Here's how the part is built. I have some questions about the finished solid (model axes, mm). A direction names the side the tool comes from. Round coordinates to 2 decimals unless told otherwise and drop trailing zeros. Loops run counter-clockwise (first coordinate to the right, second up) from the corner with the lowest first, then second, coordinate; pieces in that order, holes last. Notation, with made-up numbers: (-10, 81) -> (24, 81) arc R25 cw to (24, 116) -> close; hole circle Ø8 at (-10, 30). An arc over 180 degrees is marked (long way). Use CSV: the item, a comma, the result in double quotes. Start each with the question number.
from build123d import *

# Parameters (mm, degrees)
EXTRUDE_1_DEPTH     = 15
SKETCH_2_R          = 3.25
SKETCH_2_W          = 10
SKETCH_2_H          = 7
CUT_EXTRUDE_1_DEPTH = 37
SKETCH_3_W          = 7
SKETCH_3_H          = 25
CUT_EXTRUDE_2_DEPTH = 37
FILLET_1_R          = 2
FILLET_2_R          = 2


with BuildPart() as part:
    # 草图1 → 凸台-拉伸1 (new body)
    with BuildSketch(Plane.XY):
        Polygon((-3.257989732, 3.83894099), (16.742010268, 3.83894099), (16.742010268, 0.83894099), (-18.257989732, 0.83894099), (-18.257989732, 24.83894099), (-3.257989732, 24.83894099), align=None)
        with BuildLine():
            Line((-12.257989732, 18.83894099), (-12.257989732, 8.83894099))
            ThreePointArc((-12.257989732, 8.83894099), (-10.757989732, 7.33894099), (-9.257989732, 8.83894099))
            Line((-9.257989732, 8.83894099), (-9.257989732, 18.83894099))
            ThreePointArc((-9.257989732, 18.83894099), (-10.757989732, 20.33894099), (-12.257989732, 18.83894099))
        make_face(mode=Mode.SUBTRACT)
    extrude(amount=EXTRUDE_1_DEPTH)

    # 草图2 → 切除-拉伸1 (cut)
    with BuildSketch(Plane(origin=(0, 24.83894099, 0), x_dir=(1, 0, 0), z_dir=(0, 1, 0))):
        with Locations(Location((6.742010268, -7.5, 0), (0, 0, 180))):
            Circle(SKETCH_2_R)
        with Locations((-13.257989732, -7.5)):
            Rectangle(SKETCH_2_W, SKETCH_2_H)
    extrude(amount=-CUT_EXTRUDE_1_DEPTH, mode=Mode.SUBTRACT)

    # 草图3 → 切除-拉伸2 (cut)
    with BuildSketch(Plane(origin=(-3.257989732, 0, 0), x_dir=(0, 0, -1), z_dir=(1, 0, 0))):
        with Locations((-7.5, 12.33894099)):
            Rectangle(SKETCH_3_W, SKETCH_3_H)
    extrude(amount=-CUT_EXTRUDE_2_DEPTH, mode=Mode.SUBTRACT)

    # 圆角1
    fillet_1_edges = [part.edges().sort_by_distance(p)[0] for p in [
        (-3.257989732, 2.33894099, 11),
        (-3.257989732, 2.33894099, 4),
    ]]
    fillet(fillet_1_edges, radius=FILLET_1_R)

    # 圆角2
    fillet_2_edges = [part.edges().sort_by_distance(p)[0] for p in [
        (-3.257989732, 3.83894099, 2),
        (-3.257989732, 3.83894099, 13),
        (-4.257989732, 3.83894099, 11),
        (-4.257989732, 3.83894099, 4),
    ]]
    fillet(fillet_2_edges, radius=FILLET_2_R - 0.0001)  # a hair under: the kernel refuses the full size


solid = part.part
Q1. For faces 4 (the flat face through (-18.258, 13, 13)), 5 (the flat face through (-3.258, 2, 8)), 6 (the cylindrical face through (-10.79, 7.34, 12.97)), 7 (the flat face through (-3.258, 15, 2)), 8 (the flat face through (3, 0.839, 7)), which set-ups out of +Z, -Z, +X, -X, +Y, -Y let a thin tool reach every point of the face, with its end or its side?
Q2. Will these pins go through, and if not, where does the flat tip stop? pin 1 Ø2.5 at (y, z) = (2.5, 8) entering from -X; pin 2 Ø7.5 at (x, z) = (6, 9.5) entering from +Y; pin 3 Ø3 at (y, z) = (16, 14) entering from +X.
Q3. I want a section at D-D, the plane x = -11. List the corners of the cut face in (y, z) for me, then the cut area to 3 significant figures.
Q4. I want a section at A-A, the plane x = -6.5. List the corners of the cut face in (y, z) for me, then the cut area to 3 significant figures.
Q5. I want a section at C-C, the plane z = 2. List the corners of the cut face in (x, y) for me.
Q6. I need wall thicknesses on line 1 along Z through (x, y) = (-14.5, 19.5); line 2 along X through (y, z) = (13.25, 2.5); line 3 along Y through (x, z) = (1.5, 5). Which ranges of each line are inside material? Lowest first, please.
Q7. If we mould it in two halves opening along Y, with no side actions, what happens to faces 1 (the cylindrical face through (-10.79, 7.34, 1.97)), 2 (the flat face through (16.742, 2, 7)), 3 (the cylindrical face through (-3.29, 4.41, 4.6))? For each: pulls with the +Y half, pulls with the -Y half, needs draft (parallel to the pull), parting line crosses it, or undercut.
Q8. I want a section at B-B, the plane y = 6.25. List the corners of the cut face in (x, z) for me.
Values found:
1,face 4,"+Z, -Z, -X, +Y, -Y"
1,face 5,"-X, +Y, -Y"
1,face 6,"+Z, -Z"
1,face 7,"+Z, -Z, +X, +Y"
1,face 8,"+Z, -Z, +X, -X, -Y"
2,pin 1,"x = -3.27"
2,pin 2,"y = 3.84"
2,pin 3,"x = -3.26"
3,outline,"(0.84, 0) -> (7.36, 0) -> (7.36, 4) -> (0.84, 4) -> close; (0.84, 11) -> (7.36, 11) -> (7.36, 15) -> (0.84, 15) -> close; (20.32, 0) -> (24.84, 0) -> (24.84, 4) -> (20.32, 4) -> close; (20.32, 11) -> (24.84, 11) -> (24.84, 15) -> (20.32, 15) -> close"
3,area,"88.3 mm2"
4,outline,"(0.84, 0) -> (24.84, 0) -> (24.84, 4) -> (0.84, 4) -> close; (0.84, 11) -> (24.84, 11) -> (24.84, 15) -> (0.84, 15) -> close"
4,area,"192 mm2"
5,outline,"(-18.26, 0.84) -> (16.74, 0.84) -> (16.74, 3.84) -> (-1.26, 3.84) arc R2 cw to (-3.26, 5.84) -> (-3.26, 24.84) -> (-18.26, 24.84) -> close; hole (-12.26, 8.84) arc R1.5 ccw to (-9.26, 8.84) -> (-9.26, 18.84) arc R1.5 ccw to (-12.26, 18.84) -> close"
6,line 1,"0 to 4, 11 to 15"
6,line 2,"-18.26 to -12.26, -9.26 to -3.26"
6,line 3,"0.84 to 3.84"
7,face 1,"undercut"
7,face 2,"needs draft"
7,face 3,"pulls with the +Y half"
8,outline,"(-18.26, 0) -> (-3.26, 0) -> (-3.26, 4) -> (-18.26, 4) -> close; (-18.26, 11) -> (-3.26, 11) -> (-3.26, 15) -> (-18.26, 15) -> close"
